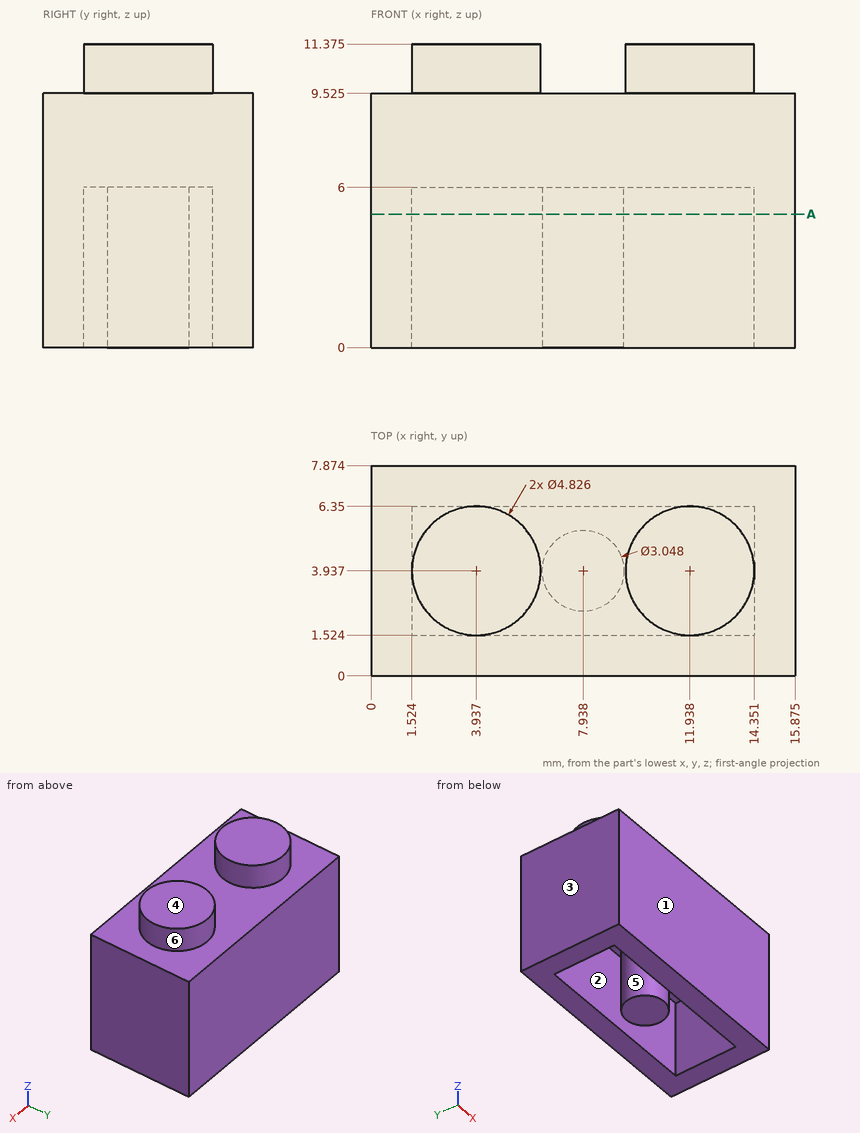
Geometry check sheet. Reference: drawing and pictorial views, mm from the part's lowest x, y, z. A direction names the side the tool comes from. Round coordinates to 2 decimals unless told otherwise and drop trailing zeros. Use a Markdown table: item, result. Add a question column.
1) Set-up check for the marked faces 4, 5 and 6: record each of +Z, -Z, +X, -X, +Y, -Y from which the full face is reachable in a straight line by a thin tool's end or side.
2) Section check A-A (z = 5). Count the separate pieces of the cut face and the enclosed holes in it.
3) Thickness scan on line 1 along Z through (x, y) = (6.5, 1.75) (1 decimal); line 2 along Z through (x, y) = (15, 3.5) (1 decimal). Record the ranges inside material, lowest first.
4) Mould release check, pull along Y, two halves, no side actions. Record for the marked faces 1, 2 and 3: released by +Y, released by -Y, zero draft, split by the parting line, or undercut.
Established:
| question | item | result |
|---|---|---|
| 1 | face 4 | +Z, +X, -X, +Y, -Y |
| 1 | face 5 | -Z |
| 1 | face 6 | +Z |
| 2 | separate pieces | 2 |
| 2 | enclosed holes | 1 |
| 3 | line 1 | 6 to 9.5 |
| 3 | line 2 | 0 to 9.5 |
| 4 | face 1 | released by -Y |
| 4 | face 2 | undercut |
| 4 | face 3 | zero draft |
